Verification items for this drawing (mm, ordinates from the low corner). Coordinates: 2 decimals unless noted, no trailing zeros. Order: outer loops, then holes, each group sorted by start corner. A loop starts at its lowest first (then second) coordinate and runs counter-clockwise, first axis right, second up. Notation, with made-up numbers: (-25.75, 89.25) -> (9.25, 89.25) arc R29 cw to (9.25, 120.25) -> close; hole circle Ø6 at (-11, 18). An arc over 180 degrees is marked (long way). Write each question's results on one line, items separated by ' | '. Start each with the question number.
(1) Thickness scan on probe 1 along Y at (x, z) = (12.7, 4.5); probe 2 along Y at (x, z) = (91, 3.75); probe 3 along X at (y, z) = (4.5, 5) (1 decimal). Record the ranges inside material, lowest first. Write a range as [from, to].
(2) Cross-section at D-D on x = 88.5. Enter the section's corners in (y, z).
(3) Cross-section at A-A on x = 12.7. Enter the section's corners in (y, z), and give its area (3 significant figures).
(4) Cross-section at B-B on y = 38.1. Give the number of separate pieces and of enclosed holes in the cut face.
(5) Go/stop test with a flat-tipped pin: pin 1 (4 mm diameter, centred on x = 25.4, y = 38.1, fed in from -Z). Record where the tip stops, or that it passes through.
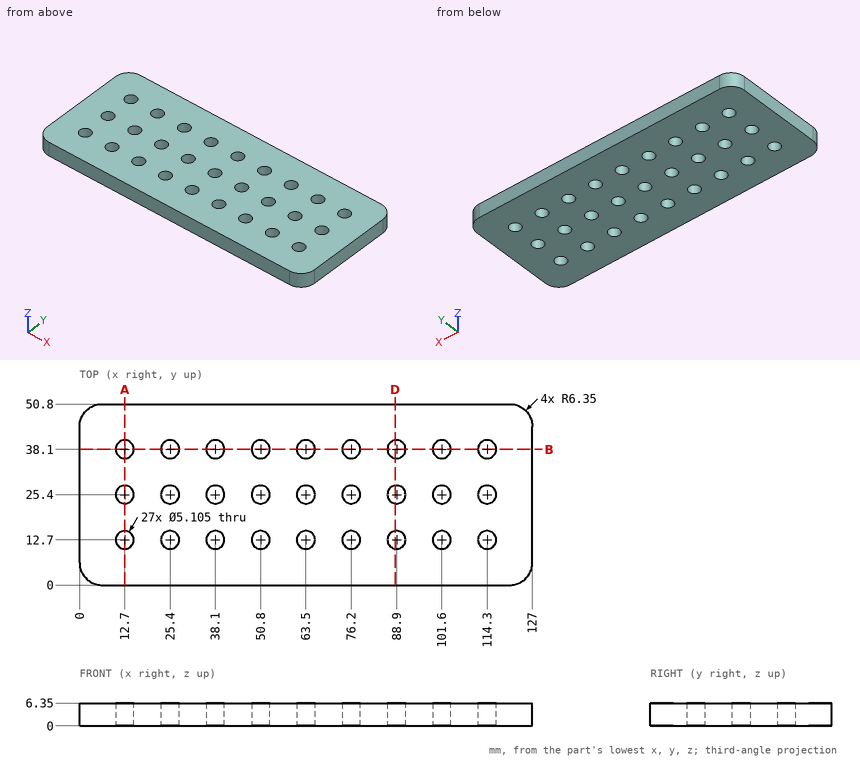
Results are:
1) probe 1: y = [0, 10.15], [15.25, 22.85], [27.95, 35.55], [40.65, 50.8] | probe 2: y = [0, 11.25], [14.15, 23.95], [26.85, 36.65], [39.55, 50.8] | probe 3: x = [0.3, 126.7]
2) outline: (0, 0) -> (10.18, 0) -> (10.18, 6.35) -> (0, 6.35) -> close; (15.22, 0) -> (22.88, 0) -> (22.88, 6.35) -> (15.22, 6.35) -> close; (27.92, 0) -> (35.58, 0) -> (35.58, 6.35) -> (27.92, 6.35) -> close; (40.62, 0) -> (50.8, 0) -> (50.8, 6.35) -> (40.62, 6.35) -> close
3) outline: (0, 0) -> (10.15, 0) -> (10.15, 6.35) -> (0, 6.35) -> close; (15.25, 0) -> (22.85, 0) -> (22.85, 6.35) -> (15.25, 6.35) -> close; (27.95, 0) -> (35.55, 0) -> (35.55, 6.35) -> (27.95, 6.35) -> close; (40.65, 0) -> (50.8, 0) -> (50.8, 6.35) -> (40.65, 6.35) -> close | area: 225 mm2
4) separate pieces: 10 | enclosed holes: 0
5) pin 1: passes through
